Geometry check sheet. Reference: the model listing, model coordinates, mm. A direction names the side the tool comes from. Round coordinates to 2 decimals unless told otherwise and drop trailing zeros. Order: outer loops, then holes, each group sorted by start corner. A loop starts at its lowest first (then second) coordinate and runs counter-clockwise, first axis right, second up.
(1) Sectioned sample at A-A (y = 0.85). Record the boundary of the cut face in (x, z), plus the area to 3 significant figures.
(2) Material ranges on line 1 along X through (y, z) = (0.3, 7.25); line 2 along Y through (x, z) = (5.85, 1); line 3 along Z through (x, y) = (4.35, 1.5), recorded low to high.
(3) Sectioned sample at C-C (z = 3.5). Record the boundary of the cut face in (x, y), plus the area to 3 significant figures.
(4) Go/stop test with flat-tipped pins: pin 1 (1.1 mm diameter, centred on x = 5, z = 2, fed in from +Y); pin 2 (0.6 mm diameter, centred on x = 4, z = 7, fed in from -Y); pin 3 (1 mm diameter, centred on x = 4, z = 2.5, fed in from -Y). Record where each tip stops, or that it passes through.
(5) Sectioned sample at D-D (x = 4.15). Record the boundary of the cut face in (y, z), plus the area to 3 significant figures.
(6) Release check for a two-part mould opening along X. For faces 5 (the face through (6, 1, 0)), 6 (the face through (6.2, 1, 4)), 7 (the face through (4, 1, 0.5)), 8 (the face through (1.5, 1, 4)) record: +X half, -X half, draft (parallel to the pull), parting line (faces both ways), or undercut.
(7) Sectioned sample at B-B (x = 5.9). Record the boundary of the cut face in (y, z), plus the area to 3 significant figures.
(8) Set-up check for faces 1 (the face through (4, 2.1, 2)), 2 (the face through (5, 1, 7)), 3 (the face through (4, 0.5, 2)), 4 (the face through (2, 1, 7)): record each of +Z, -Z, +X, -X, +Y, -Y from which the full face is reachable in a straight line by a thin tool's end or side.
Autodesk Inventor part; units mm, degrees
ref_plane "Płaszczyzna konstrukcyjna1" through (-1, -0.5, 6.4) normal (0, 0, -1) x (0, 1, 0)
ref_plane "YZ Plane" through (0, 0, 0) normal (1, 0, 0) x (0, 1, 0)
ref_plane "XZ Plane" through (0, 0, 0) normal (0, 1, 0) x (-1, 0, 0)
sketch "Szkic1" plane through (0, 0, 0) normal (0, 0, 1) x (1, 0, 0)
  line L0 (2.7, 2.2) -> (2.7, 0.4)
  line L1 (5, 0.4) -> (5, 2.2)
  line L2 (5, 2.2) -> (5, 2.6)
  line L3 (2.7, 2.6) -> (2.7, 2.2)
  line L4 (2.7, 0.4) -> (2.7, 0)
  line L5 (5, 0) -> (5, 0.4)
  line L6 (2.7, 0) -> (5, 0)
  line L7 (5, 2.6) -> (2.7, 2.6)
  line L8 (2.5, -0.2) -> (2.5, 0.4)
  line L9 (2.5, 0.4) -> (2.5, 2.2)
  line L10 (2.5, 2.2) -> (2.5, 2.8)
  line L11 (2.5, 2.8) -> (5.2, 2.8)
  line L12 (5.2, 2.8) -> (5.2, 2.2)
  line L13 (5.2, 2.2) -> (5.2, 0.4)
  line L14 (5.2, 0.4) -> (5.2, -0.2)
  line L15 (5.2, -0.2) -> (2.5, -0.2)
  line L16 (2.7, 0) -> (2.7, 2.6)
  line L17 (0, 2.6) -> (2.7, 2.6)
  line L18 (0, 0) -> (0, 2.6)
  line L19 (0, 0) -> (2.7, 0)
  line L20 (5, 2.6) -> (5, 0)
  line L21 (5, 0) -> (10, 0)
  line L22 (10, 0) -> (10, 2.6)
  line L23 (5, 2.6) -> (10, 2.6)
  line L24 (2.5, 0) -> (1.5, 0)
  line L25 (1.5, 0) -> (1.5, 2.6)
  line L26 (1.5, 2.6) -> (2.5, 2.6)
  line L27 (2.5, 2.6) -> (2.5, 0)
  line L28 (5.2, 0) -> (6.2, 0)
  line L29 (6.2, 0) -> (6.2, 2.6)
  line L30 (6.2, 2.6) -> (5.2, 2.6)
  line L31 (5.2, 2.6) -> (5.2, 0)
  dimension "d0" = 0.2
  dimension "d1" = 1
  dimension "d2" = 1
extrude "Wyciągnięcie proste1" add sketch "Szkic1" along normal blind 0.5 contours L10 L9 L8 L19 L25 L17 | L23 L29 L21 L14 L13 L12
sketch "Szkic2" plane through (0, 0, 0.5) normal (0, 0, 1) x (1, 0, 0)
  line L0 (1.5, 0) -> (2.5, 0)
  line L1 (2.5, 0) -> (2.5, 2.6)
  line L2 (2.5, 2.6) -> (1.5, 2.6)
  line L3 (1.5, 2.6) -> (1.5, 0)
  line L4 (6.2, 2.6) -> (5.2, 2.6)
  line L5 (5.2, 2.6) -> (5.2, 0)
  line L6 (5.2, 0) -> (6.2, 0)
  line L7 (6.2, 0) -> (6.2, 2.6)
  line L8 (1.5, 2.6) -> (6.2, 2.6)
  line L9 (6.2, 2.6) -> (6.2, 0)
  line L10 (6.2, 0) -> (1.5, 0)
  line L11 (1.5, 0) -> (1.5, 2.6)
  point P0 (0, 0)
ref_plane "Płaszczyzna konstrukcyjna1" through (-1, -0.5, 6.4) normal (0, 0, -1) x (0, 1, 0)
extrude "Wyciągnięcie proste2" add sketch "Szkic2" along normal up to surface (5.9 mm away)
sketch "Szkic3" plane through (1.5, 0, 6.4) normal (0, 0, 1) x (1, 0, 0)
  line L0 (9.5, 3.1) -> (-2.5, 3.1)
  line L1 (-2.5, 3.1) -> (-2.5, -0.5)
  line L2 (-2.5, -0.5) -> (9.5, -0.5)
  line L3 (9.5, -0.5) -> (9.5, 3.1)
  line L4 (0, 2.6) -> (0, 0)
  line L5 (0, 0) -> (4.7, 0)
  line L6 (4.7, 0) -> (4.7, 2.6)
  line L7 (4.7, 2.6) -> (0, 2.6)
  line L8 (0, 3.1) -> (4.7, 3.1)
  line L9 (4.7, 3.1) -> (4.7, -0.5)
  line L10 (4.7, -0.5) -> (0, -0.5)
  line L11 (0, -0.5) -> (0, 3.1)
  line L12 (-2.4, 3) -> (9.4, 3)
  line L13 (9.4, 3) -> (9.4, -0.4)
  line L14 (9.4, -0.4) -> (-2.4, -0.4)
  line L15 (-2.4, -0.4) -> (-2.4, 3)
  point P0 (-1.5, 0)
  point P1 (4.7, 3)
  point P2 (0, 3)
  point P3 (0, -0.4)
  point P4 (4.7, -0.4)
  dimension "d7" = 0.1
extrude "Wyciągnięcie proste3" add sketch "Szkic3" against normal blind 1 contours L9 L7 L11 L12 | L6 L5 L4 L7 | L14 L11 L5 L9
sketch "Szkic4" plane through (1.5, -0.4, 6.4) normal (0, 0, 1) x (1, 0, 0)
  line L0 (-2.2, 3.2) -> (9.2, 3.2)
  line L1 (9.2, 0.2) -> (-2.2, 0.2)
  line L2 (-2.2, 0.2) -> (-2.2, 3.2)
  line L3 (9.2, 3.2) -> (9.2, 0.2)
  line L4 (0, 3.4) -> (0, 0)
  line L5 (0, 0) -> (4.7, 0)
  line L6 (4.7, 0) -> (4.7, 3.4)
  line L7 (4.7, 3.4) -> (0, 3.4)
  line L8 (0.5, 0.5) -> (0.5, 2.9)
  line L9 (0.5, 2.9) -> (4.2, 2.9)
  line L10 (4.2, 2.9) -> (4.2, 0.5)
  line L11 (4.2, 0.5) -> (0.5, 0.5)
  line L12 (1, 0.4) -> (1, 3)
  line L13 (0.5, 2.9) -> (1, 2.9)
  line L14 (1, 2.9) -> (1, 0.5)
  line L15 (1, 0.5) -> (0.5, 0.5)
  line L16 (0.5, 0.5) -> (0.5, 2.9)
  line L17 (1.5, 2.9) -> (1.5, 0.5)
  line L18 (2, 2.9) -> (2, 0.5)
  line L19 (2.5, 2.9) -> (2.5, 0.5)
  line L20 (3, 2.9) -> (3, 0.5)
  line L21 (3.5, 2.9) -> (3.5, 0.5)
  line L22 (4, 2.9) -> (4, 0.5)
  point P0 (-1.5, 0.4)
  point P1 (4, 0.5)
  point P2 (4, 2.9)
  point P3 (3.5, 2.9)
  point P4 (3.5, 0.5)
  point P5 (3, 0.5)
  point P6 (3, 2.9)
  point P7 (2.5, 0.5)
  point P8 (2, 0.5)
  point P9 (1.5, 2.9)
  point P10 (1.5, 0.5)
  point P11 (1, 2.9)
  dimension "d10" = 0.5
  dimension "d13" = 0.5
extrude "Wyciągnięcie proste4" add sketch "Szkic4" along normal blind 0.9 contours L8 L9 L12 L11 | L17 L9 L18 L11 | L19 L9 L20 L11 | L21 L9 L22 L11
sketch "Szkic5" plane through (1.5, 0, 0) normal (0, -1, 0) x (1, 0, 0)
  line L0 (4.7, 5.4) -> (0, 5.4)
  line L1 (0, 0) -> (0, 5.4)
  line L2 (0, 0) -> (1, 0)
  line L3 (1, 0) -> (1, 0.5)
  line L4 (1, 0.5) -> (3.7, 0.5)
  line L5 (3.7, 0) -> (3.7, 0.5)
  line L6 (3.7, 0) -> (4.7, 0)
  line L7 (4.7, 0) -> (4.7, 5.4)
  point P0 (-1.5, 0)
extrude "Wyciągnięcie proste5" cut sketch "Szkic5" against normal blind 0.5
sketch "Szkic6" plane through (5.2, 2.6, 0) normal (0, 1, 0) x (1, 0, 0)
  line L0 (-3.7, -5.4) -> (1, -5.4)
  line L1 (1, 0) -> (1, -5.4)
  line L2 (1, 0) -> (0, 0)
  line L3 (0, 0) -> (0, -0.5)
  line L4 (0, -0.5) -> (-2.7, -0.5)
  line L5 (-2.7, 0) -> (-2.7, -0.5)
  line L6 (-2.7, 0) -> (-3.7, 0)
  line L7 (-3.7, 0) -> (-3.7, -5.4)
  point P0 (-5.2, 0)
extrude "Wyciągnięcie proste6" cut sketch "Szkic6" against normal blind 0.5
fillet "Zaokrąglenie1" radius 2 2 edges at (3.85, 2.1, 5.4) (3.85, 0.5, 5.4)
properties part number "wlacznik_2"
Answer below:
1. outline: (1.5, 0) - (2.5, 0) - (2.5, 0.5) - (5.2, 0.5) - (5.2, 0) - (6.2, 0) - (6.2, 6.4) - (5.5, 6.4) - (5.5, 7.3) - (5, 7.3) - (5, 6.4) - (4.5, 6.4) - (4.5, 7.3) - (4, 7.3) - (4, 6.4) - (3.5, 6.4) - (3.5, 7.3) - (3, 7.3) - (3, 6.4) - (2.5, 6.4) - (2.5, 7.3) - (2, 7.3) - (2, 6.4) - (1.5, 6.4) - close
1. area: 30.5 mm2
2. line 1: x = 2 to 2.5, 3 to 3.5, 4 to 4.5, 5 to 5.5
2. line 2: y = 0.5 to 2.1
2. line 3: z = 0.5 to 7.3
3. outline: (1.5, 0.5) - (6.2, 0.5) - (6.2, 2.1) - (1.5, 2.1) - close
3. area: 7.52 mm2
4. pin 1: stops at y = 2.1
4. pin 2: stops at y = 0.1
4. pin 3: stops at y = 0.5
5. outline: (-0.4, 5.4) arc R2 cw to (0.5, 3.73) - (0.5, 0.5) - (2.1, 0.5) - (2.1, 3.73) arc R2 cw to (3, 5.4) - (3, 6.4) - (2.5, 6.4) - (2.5, 7.3) - (0.1, 7.3) - (0.1, 6.4) - (-0.4, 6.4) - close
5. area: 14.3 mm2
6. face 5: draft
6. face 6: +X half
6. face 7: undercut
6. face 8: -X half
7. outline: (-0.4, 5.4) arc R2 cw to (0.5, 3.73) - (0.5, 0) - (2.1, 0) - (2.1, 3.73) arc R2 cw to (3, 5.4) - (3, 6.4) - (-0.4, 6.4) - close
7. area: 12.9 mm2
8. face 1: -Z, +X, -X, +Y
8. face 2: +Z, +Y, -Y
8. face 3: -Z, +X, -X, -Y
8. face 4: +Z, -X, +Y, -Y
